Build history of the part. All positions in model axes, mm. Round coordinates to 2 decimals unless told otherwise and drop trailing zeros. Loops run counter-clockwise (first coordinate to the right, second up) from the corner with the lowest first, then second, coordinate; pieces in that order, holes last. Notation, with made-up numbers: (56, 9.5) - (73, 9.5) arc R18 ccw to (73, 43.5) - close; hole circle Ø10 at (-22.5, 30). An arc over 180 degrees is marked (long way). One line per question, with ' | ' between items. Start each with the question number.
from build123d import *

# Parameters (mm, degrees)
ESQUISSE1_R             = 9.525
BOSS_EXTRU_1_DEPTH      = 5.08
ESQUISSE2_R             = 2
ESQUISSE2_R_2           = 2.5
ENL_V_MAT_EXTRU_1_DEPTH = 15.396445742


with BuildPart() as part:
    # Esquisse1 → Boss.-Extru.1 (new body)
    with BuildSketch(Plane(origin=(0, 0, 0), x_dir=(1, 0, 0), z_dir=(0, 1, 0))):
        with Locations(Location((0, 0, 0), (0, 0, 270))):
            Circle(ESQUISSE1_R)
    extrude(amount=BOSS_EXTRU_1_DEPTH)

    # Esquisse2 → Enlèv. mat.-Extru.1 (cut, through all)
    with BuildSketch(Plane(origin=(0, 5.08, 0), x_dir=(1, 0, 0), z_dir=(0, 1, 0))):
        with Locations(Location((0, 6.35, 0), (0, 0, 270))):
            Circle(ESQUISSE2_R)
        with Locations(Location((-6.35, 0, 0), (0, 0, 270))):
            Circle(ESQUISSE2_R)
        with Locations(Location((6.35, 0, 0), (0, 0, 270))):
            Circle(ESQUISSE2_R)
        with Locations(Location((0, -6.35, 0), (0, 0, 270))):
            Circle(ESQUISSE2_R)
        with Locations(Location((0, 0, 0), (0, 0, 270))):
            Circle(ESQUISSE2_R_2)
    extrude(amount=-ENL_V_MAT_EXTRU_1_DEPTH, mode=Mode.SUBTRACT)


solid = part.part
1) Wall check: line 1 (X direction, y = 2.1, z = 0) (3 decimals); line 2 (Z direction, x = 1.75, y = 3.35); line 3 (Z direction, x = 1, y = 0.9). Give the ranges that are in metal, low to high. Write a range as [from, to].
2) Two-plate mould, pull along X, no slides. Class faces 1 (the cylindrical face through (-1.217, 2.576, 4.763)), 2 (the cylindrical face through (-5.796, 2.504, -7.559)), 3 (the flat face through (-2, 0, 2)): +X half, -X half, draft (parallel to the pull), parting line (faces both ways), or undercut.
3) Saw through at D-D on z = -6.35. Write the cut outline in (x, y), and give its area (3 significant figures).
4) Drop a flat-ended pin along its axis: pin 1 (1.5 mm diameter, centred on y = 1, z = -7.5, fed in from +X). Give the stop position or say it passes through.
5) Saw through at A-A on x = 0. Write the cut outline in (y, z) (3 decimals), and give its area (3 significant figures).
6) Saw through at C-C on x = 6.35. Write the cut outline in (y, z), and give its area (3 significant figures).
7) Saw through at B-B on z = 0. Write the cut outline in (x, y) (3 decimals), and give its area (3 significant figures).
Answer key:
1) line 1: [-9.525, -8.35], [-4.35, -2.5], [2.5, 4.35], [8.35, 9.525] | line 2: [-9.36, -7.32], [-5.38, -1.79], [1.79, 5.38], [7.32, 9.36] | line 3: [-9.47, -8.08], [-4.62, -2.29], [2.29, 4.62], [8.08, 9.47]
2) face 1: undercut | face 2: parting line | face 3: draft
3) outline: (-7.1, 0) - (-2, 0) - (-2, 5.08) - (-7.1, 5.08) - close; (2, 0) - (7.1, 0) - (7.1, 5.08) - (2, 5.08) - close | area: 51.8 mm²
4) pin 1: x = 6.72
5) outline: (0, -9.525) - (5.08, -9.525) - (5.08, -8.35) - (0, -8.35) - close; (0, -4.35) - (5.08, -4.35) - (5.08, -2.5) - (0, -2.5) - close; (0, 2.5) - (5.08, 2.5) - (5.08, 4.35) - (0, 4.35) - close; (0, 8.35) - (5.08, 8.35) - (5.08, 9.525) - (0, 9.525) - close | area: 30.7 mm²
6) outline: (0, -7.1) - (5.08, -7.1) - (5.08, -2) - (0, -2) - close; (0, 2) - (5.08, 2) - (5.08, 7.1) - (0, 7.1) - close | area: 51.8 mm²
7) outline: (-9.525, 0) - (-8.35, 0) - (-8.35, 5.08) - (-9.525, 5.08) - close; (-4.35, 0) - (-2.5, 0) - (-2.5, 5.08) - (-4.35, 5.08) - close; (2.5, 0) - (4.35, 0) - (4.35, 5.08) - (2.5, 5.08) - close; (8.35, 0) - (9.525, 0) - (9.525, 5.08) - (8.35, 5.08) - close | area: 30.7 mm²
